Study the drawing (mm; zero at the part's minimum x, y, z) and answer. A direction names the side the tool comes from. Coordinates: 2 decimals unless noted, no trailing zeros. Order: outer loops, then holes, each group sorted by start corner. A loop starts at its lowest first (then second) coordinate and runs counter-clockwise, first axis right, second up. Notation, with made-up numbers: (66, 67.25) -> (78, 67.25) arc R24 ccw to (78, 94.25) -> close; hole circle Ø2 at (67.25, 60). An arc over 180 degrees is marked (long way). Answer as CSV lines item,"result". Start each with the question number.
Item 1: Section A-A (y = 13.5) is taken. Write down the section's boundary in (x, z), then the cut area to 3 significant figures.
Item 2: Each of these flat-tipped pins is pushed along its axis until it touches: pin 1 Ø2 at (x, z) = (11.5, 10.5) entering from +Y; pin 2 Ø3 at (y, z) = (13.5, 11) entering from +X; pin 3 Ø2 at (x, z) = (11.5, 4.5) entering from +Y. Where does it stop, or does it pass through?
Item 3: Section B-B (x = 13.5) is taken. Write down the section's boundary in (y, z), then the cut area to 3 significant figures.
Item 4: Which of the six approach directions +Z, -Z, +X, -X, +Y, -Y give full straight-line access (tool end or side, diameter ignored) to the marked faces 1 and 2?
Item 5: For a pull along Y with two mould halves and no side action, classify the marked faces 3, 4 and 5 as pulls with the +Y half, pulls with the -Y half, needs draft (parallel to the pull), parting line crosses it, or undercut.
Item 6: Section D-D (y = 22.75) is taken. Write down the section's boundary in (x, z), then the cut area to 3 significant figures.
Item 7: Section C-C (z = 11) is taken. Write down the section's boundary in (x, y), then the cut area to 3 significant figures.
Item 8: Straight lines are drawn through the part: L1, parallel to Y at x = 13.5, z = 4.7; L2, parallel to Z at x = 16.8, y = 13.5; L3, parallel to Z at x = 23.5, y = 10.75. For each, find the intervals that lie inside material, in ascending order.
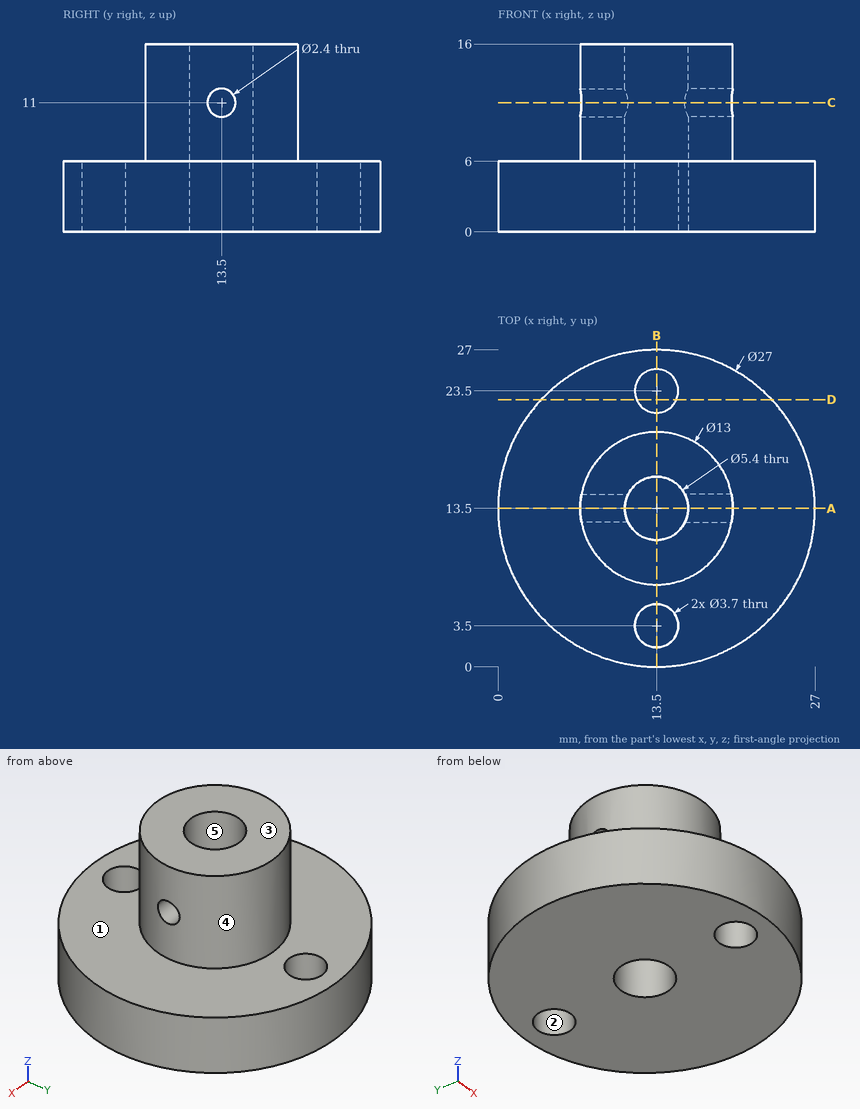
Checked values:
1,outline,"(0, 0) -> (10.8, 0) -> (10.8, 9.8) -> (7, 9.8) -> (7, 6) -> (0, 6) -> close; (7, 12.2) -> (10.8, 12.2) -> (10.8, 16) -> (7, 16) -> close; (16.2, 0) -> (27, 0) -> (27, 6) -> (20, 6) -> (20, 9.8) -> (16.2, 9.8) -> close; (16.2, 12.2) -> (20, 12.2) -> (20, 16) -> (16.2, 16) -> close"
1,area,"187 mm^2"
2,pin 1,"stops at y = 19.92"
2,pin 2,"stops at x = 20"
2,pin 3,"stops at y = 26.96"
3,outline,"(0, 0) -> (1.65, 0) -> (1.65, 6) -> (0, 6) -> close; (5.35, 0) -> (10.8, 0) -> (10.8, 16) -> (7, 16) -> (7, 6) -> (5.35, 6) -> close; (16.2, 0) -> (21.65, 0) -> (21.65, 6) -> (20, 6) -> (20, 16) -> (16.2, 16) -> close; (25.35, 0) -> (27, 0) -> (27, 6) -> (25.35, 6) -> close"
3,area,"161 mm^2"
4,face 1,"+Z"
4,face 2,"+Z, -Z"
5,face 3,"needs draft"
5,face 4,"parting line crosses it"
5,face 5,"undercut"
6,outline,"(3.67, 0) -> (11.81, 0) -> (11.81, 6) -> (3.67, 6) -> close; (15.19, 0) -> (23.33, 0) -> (23.33, 6) -> (15.19, 6) -> close"
6,area,"97.7 mm^2"
7,outline,"(7.11, 12.3) arc R6.5 ccw to (19.89, 12.3) -> (15.92, 12.3) arc R2.7 cw to (11.08, 12.3) -> close; (7.11, 14.7) -> (11.08, 14.7) arc R2.7 cw to (15.92, 14.7) -> (19.89, 14.7) arc R6.5 ccw to start"
7,area,"91.3 mm^2"
8,L1,"y = 0 to 1.65, 5.35 to 10.8, 16.2 to 21.65, 25.35 to 27"
8,L2,"z = 0 to 9.8, 12.2 to 16"
8,L3,"z = 0 to 6"
